Can you work these out from the model? Positions are in its coordinate system, mm. Face numbers are marked on the shaded views. A direction names the side the tool comes from. Coordinates: 2 decimals unless noted, no trailing zeros. Order: outer loops, then holes, each group sorted by start corner. A loop starts at its lowest first (then second) coordinate and runs counter-clockwise, first axis right, second up. Notation, with made-up numbers: (34.5, 1) -> (43.5, 1) arc R13 cw to (43.5, 12) -> close; hole circle Ø6 at (-4.5, -13.5). An arc over 180 degrees is marked (long way). Write item = value, one per line.
Autodesk Inventor part; units mm, degrees
ref_plane "Plano de trabajo2" through (-10, 12, 4) normal (1, 0, 0) x (0, 0, -1)
ref_plane "YZ Plane" through (0, 0, 0) normal (1, 0, 0) x (0, 1, 0)
ref_plane "XZ Plane" through (0, 0, 0) normal (0, 1, 0) x (-1, 0, 0)
sketch "Boceto5" plane through (-24, -1, 0) normal (0, 0, -1) x (-1, 0, 0)
  line L0 (-28, 35) -> (0, 35)
  line L1 (0, 35) -> (0, -3)
  line L2 (0, -3) -> (-28, -3)
  line L3 (-28, -3) -> (-28, 35)
  point P0 (-24, 1)
  point P1 (0, 0)
  dimension "d3" = 28
  dimension "d4" = 3
  dimension "d5" = 35
extrude "Extrusión2" add sketch "Boceto5" against normal blind 4
fillet "Empalme1" radius 3 4 edges at (-24, -4, 2) (4, -4, 2) (4, 34, 2) (-24, 34, 2)
sketch "Boceto6" plane through (-24, -1, 4) normal (0, 0, 1) x (1, 0, 0)
  line L0 (25, 35) -> (3, 35) construction
  line L1 (0, 32) -> (0, 0) construction
  point P0 (24, 1)
  point P1 (4, 31)
  dimension "d9" = 4
  dimension "d10" = 4
hole "Agujero1" at (-20, 30, 4) direction (0, 0, -1) diameter 3 end through all counterbore diameter 4 counterbore depth 2
pattern_linear "Patrón rectangular1" count 2 spacing 20 along (1, 0, 0) count 2 spacing 30 along (0, -1, 0) of "Agujero1"
sketch "Boceto7" plane through (-24, -1, 0) normal (0, 0, -1) x (-1, 0, 0)
  line L0 (-3, 35) -> (-25, 35)
  line L1 (-28, 32) -> (-28, 0)
  point P0 (-24, 1)
  point P1 (-14, 15)
  dimension "d24" = 20
  dimension "d25" = 14
hole "Agujero2" at (-10, 14, 0) direction (0, 0, 1) diameter 6 end through all
sketch "Boceto8" plane through (-24, -1, 4) normal (0, 0, 1) x (1, 0, 0)
  line L0 (5.5, 17) -> (22.5, 17)
  line L1 (22.5, 17) -> (22.5, 13)
  line L2 (22.5, 13) -> (5.5, 13)
  line L3 (5.5, 13) -> (5.5, 17)
  circle A0 centre (14, 15) radius 3
  line L4 (5.5, 17) -> (22.5, 13) construction
  line L5 (22.5, 17) -> (5.5, 13) construction
  point P0 (24, 1)
  point P1 (11.7639, 13)
  point P2 (11.7639, 17)
  point P3 (16.2361, 17)
  point P4 (16.2361, 13)
  dimension "d33" = 17
  dimension "d34" = 4
extrude "Extrusión3" cut sketch "Boceto8" against normal blind 2 contours L0 A0 L2 L3 | L0 L1 L2 A0
sketch "Boceto9" plane through (-24, -1, 4) normal (0, 0, 1) x (1, 0, 0)
  line L0 (11.7639, 13) -> (5.5, 13) construction
  line L1 (10.5, 13) -> (11.75, -1.5)
  line L2 (11.75, -1.5) -> (16.25, -1.5)
  line L3 (16.25, -1.5) -> (17.5, 13)
  line L4 (17.5, 13) -> (10.5, 13)
  line L5 (0, 32) -> (0, 0)
  point P0 (24, 1)
  dimension "d37" = 14.5
  dimension "d38" = 4.5
  dimension "d39" = 10.5
  dimension "d40" = 7
  dimension "d41" = 1.25
extrude "Extrusión4" cut sketch "Boceto9" against normal blind 2
sketch "Boceto11" plane through (-24, -1, 4) normal (0, 0, 1) x (1, 0, 0)
  line L0 (5.5, 17) -> (11.7639, 17) construction
  line L1 (10.5, 17) -> (17.5, 17)
  line L2 (17.5, 17) -> (16.25, 33.5)
  line L3 (16.25, 33.5) -> (11.75, 33.5)
  line L4 (11.75, 33.5) -> (10.5, 17)
  point P0 (24, 1)
  dimension "d44" = 16.5
  dimension "d46" = 5
  dimension "d47" = 1.25
  dimension "d48" = 7
extrude "Extrusión5" cut sketch "Boceto11" against normal blind 2
sketch "Boceto15" plane through (-13.8306, 0.9703, 10) normal (0, 0, 1) x (1, 0, 0)
  circle A0 centre (17.3236, 13.0832) radius 22.3484 construction
  circle A1 centre (4.7289, 20.1353) radius 7.5795 construction
  circle A2 centre (10.4075, 15.4052) radius 15.0152 construction
  arc A3 (-3.6953, 20.6765) -> (-5.0248, 13.0297) centre (17.3236, 13.0832) ccw
  arc A4 (-1.0419, 25.1821) -> (-3.6953, 20.6765) centre (10.4075, 15.4052) ccw
  arc A5 (1.2391, 26.9612) -> (-1.0419, 25.1821) centre (4.7289, 20.1353) ccw
  circle A6 centre (3.8306, 13.0297) radius 3 construction
  line L0 (3.8306, 13.0297) -> (-5.0248, 13.0297) construction
  line L1 (3.8306, 11.0151) -> (-6.9515, 11.0151) construction
  arc A7 (-5.5863, 21.3713) -> (-6.9515, 11.0151) centre (17.3236, 13.0832) ccw
  arc A8 (-2.5664, 26.4991) -> (-5.5863, 21.3713) centre (10.4075, 15.4052) ccw
  arc A9 (-0.3913, 28.3513) -> (-2.5664, 26.4991) centre (4.7289, 20.1353) ccw
  line L2 (0.3306, 15.0297) -> (1.5806, 31.5297) construction
  arc A10 (1.2648, 27.3612) -> (-0.3913, 28.3513) centre (0.1824, 27.4308) ccw
  line L3 (1.2648, 27.3612) -> (1.2391, 26.9612)
  arc A11 (-5.0248, 13.0297) -> (-3.6953, 5.3829) centre (17.3236, 12.9762) ccw
  arc A12 (-3.6953, 5.3829) -> (-1.0419, 0.8774) centre (10.4075, 10.6542) ccw
  arc A13 (-1.0419, 0.8774) -> (1.2391, -0.9018) centre (4.7289, 5.9242) ccw
  line L4 (3.8306, 15.0443) -> (-6.9515, 15.0443) construction
  arc A14 (-6.9515, 15.0443) -> (-5.5863, 4.6881) centre (17.3236, 12.9762) ccw
  arc A15 (-5.5863, 4.6881) -> (-2.5664, -0.4397) centre (10.4075, 10.6542) ccw
  arc A16 (-2.5664, -0.4397) -> (-0.3913, -2.2919) centre (4.7289, 5.9242) ccw
  arc A17 (-0.3913, -2.2919) -> (1.2648, -1.3018) centre (0.1824, -1.3713) ccw
  line L5 (1.2648, -1.3018) -> (1.2391, -0.9018)
  point P0 (13.8306, -0.9703)
  point P1 (0.3306, 11.0297)
  point P2 (-7.0394, 13.0297)
  dimension "d51" = 20
  dimension "d52" = 20
  dimension "d53" = 21.75
  dimension "d55" = 1.9267
  dimension "d56" = 0.4
extrude "Extrusión6" add sketch "Boceto15" against normal blind 6
ref_plane "Plano de trabajo2" through (-10, 12, 4) normal (1, 0, 0) x (0, 0, -1)
mirror "Simetría2" about plane through (-10, 12, 4) normal (1, 0, 0) of "Extrusión6"
properties part number "base"
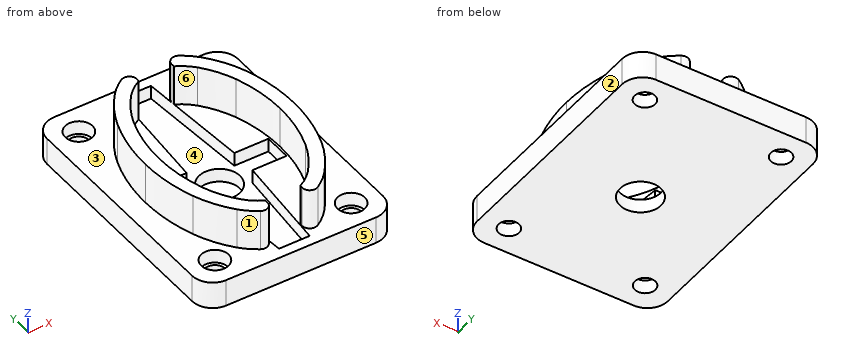
Item 1: I want a section at B-B, the plane x = -11. Please give me the cut outline in (y, z), plus the area to 3 significant figures.
A:
outline = (-4, 0) -> (11.17, 0) -> (11.17, 2) -> (-2.5, 2) -> (-2.5, 4) -> (-4, 4) -> close; (16.83, 0) -> (34, 0) -> (34, 4) -> (32.5, 4) -> (32.5, 2) -> (16.83, 2) -> close
area = 70.7 mm2
Item 2: I want a section at C-C, the plane y = 11.5. Please give me the cut outline in (x, z).
A:
outline = (-24, 0) -> (-11.66, 0) -> (-11.66, 2) -> (-13.46, 2) -> (-13.46, 4) -> (-18.72, 4) -> (-18.72, 10) -> (-20.75, 10) -> (-20.75, 4) -> (-24, 4) -> close; (-8.34, 0) -> (4, 0) -> (4, 4) -> (0.75, 4) -> (0.75, 10) -> (-1.28, 10) -> (-1.28, 4) -> (-6.54, 4) -> (-6.54, 2) -> (-8.34, 2) -> close
Item 3: If we mould it in two halves opening along X, with no side actions, what happens to the marked faces 1, 2, 3 and 4? For each: pulls with the +X half, pulls with the -X half, needs draft (parallel to the pull), parting line crosses it, or undercut.
A:
face_1 = pulls with the -X half
face_2 = pulls with the +X half
face_3 = undercut
face_4 = undercut
Item 4: For the marked faces 5 and 6, which set-ups out of +Z, -Z, +X, -X, +Y, -Y let a thin tool reach every point of the face, with its end or its side?
A:
face_5 = +Z, -Z, +X, -X, -Y
face_6 = +Z
Item 5: I want a section at D-D, the plane x = 0. Please give me the cut outline in (y, z).
A:
outline = (-4, 0) -> (-1.5, 0) -> (-1.5, 2) -> (-2, 2) -> (-2, 4) -> (-4, 4) -> close; (1.5, 0) -> (28.5, 0) -> (28.5, 2) -> (28, 2) -> (28, 4) -> (20.51, 4) -> (20.51, 10) -> (7.49, 10) -> (7.49, 4) -> (2, 4) -> (2, 2) -> (1.5, 2) -> close; (31.5, 0) -> (34, 0) -> (34, 4) -> (32, 4) -> (32, 2) -> (31.5, 2) -> close
Item 6: I want a section at A-A, the plane z = 3.25. Please give me the cut outline in (x, y), plus the area to 3 significant figures.
A:
outline = (-24, -1) arc R3 ccw to (-21, -4) -> (1, -4) arc R3 ccw to (4, -1) -> (4, 31) arc R3 ccw to (1, 34) -> (-21, 34) arc R3 ccw to (-24, 31) -> close; hole circle Ø4 at (-20, 0); hole circle Ø4 at (-20, 30); hole (-18.5, 12) -> (-13.5, 12) -> (-12.25, -2.5) -> (-7.75, -2.5) -> (-6.5, 12) -> (-1.5, 12) -> (-1.5, 16) -> (-6.5, 16) -> (-7.75, 32.5) -> (-12.25, 32.5) -> (-13.5, 16) -> (-18.5, 16) -> close; hole circle Ø4 at (0, 0); hole circle Ø4 at (0, 30)
area = 760 mm2
Item 7: I'm going to push flat-ended pins straight in: P1, Ø1.5, axis at x = -11.5, y = 25.5, coming from the +Z side; P2, Ø6, axis at y = 8.5, z = 7.5, coming from the -X side. Where does each tip first touch, or does it pass through?
A:
P1 = 2
P2 = -20.75
Item 8: If I drill on probe 1 along Y at (x, z) = (-20, 2.5); probe 2 along X at (y, z) = (0, 1.2); probe 3 along Y at (x, z) = (0, 0.9), over which ranges is the centre line in solid material (lowest first)?
A:
probe_1 = -4 to -2, 2 to 28, 32 to 34
probe_2 = -24 to -21.5, -18.5 to -1.5, 1.5 to 4
probe_3 = -4 to -1.5, 1.5 to 28.5, 31.5 to 34
